Model file for the job. Use its own axes, mm. A direction names the side the tool comes from. Give positions to 0.01 mm unless a question says otherwise; leave off trailing zeros. Write each loop counter-clockwise with the first axis right and the second up, starting at its lowest first coordinate (ties: lowest second). Pieces come first, ordered by that corner, then holes. Notation, with made-up numbers: (86, -28) - (103, -28) arc R12 ccw to (103, -15) - close; hole circle Ø7 at (-10, -12.5). An arc over 180 degrees is marked (long way). One line per item, written item: value. Start each with the question number.
(1) 3-axis set-ups, long thin cutter, end or side, ignore diameter. For faces 5 (the face through (-2.685, -34.419, 0.426)), 6 (the face through (2.215, -24, 2)): which of +Z, -Z, +X, -X, +Y, -Y reach the whole face in a straight line?
(2) Cut at C-C, the plane y = -40.5. List the corners of the cut face in (x, z).
(3) Drop flat-ended pins along their axis: P1, Ø0.9, axis at y = -34.426, z = 1.5, coming from the -X side; P2, Ø1.4, axis at y = -14.426, z = 1.5, coming from the -X side. Give the stop position or say it passes through.
(4) Cut at B-B, the plane z = 0.35. State how many separate pieces and enclosed holes the cut face has, and give its area (3 significant figures).
(5) Probe L1, parallel to Y at x = -1.9, z = 1.5; L2, parallel to Y at x = 5, z = 1; L3, parallel to Y at x = -0.75, z = 1.9. List the from-to ranges inside material, lowest first.
(6) Cut at A-A, the plane y = -22. List the corners of the cut face in (x, z).
(7) Mould opens along Z. For faces 1 (the face through (1.904, -14.559, 1.471)), 2 (the face through (-2.785, -9, 1)), 3 (the face through (0, -24, 3)), 4 (the face through (-0.605, -35.203, 1.398)) say: pulls with the +Z half, pulls with the -Z half, needs draft (parallel to the pull), parting line crosses it, or undercut.
Autodesk Inventor part; units mm, degrees
ref_plane "YZ Plane" through (0, 0, 0) normal (1, 0, 0) x (0, 1, 0)
ref_plane "XZ Plane" through (0, 0, 0) normal (0, 1, 0) x (-1, 0, 0)
ref_plane "XY Plane" through (0, 0, 0) normal (0, 0, 1) x (1, 0, 0)
sketch "スケッチ1" plane through (0, 0, 0) normal (0, 0, 1) x (1, 0, 0)
  line L0 (22.7151, -43.926) -> (22.7151, -4.926) construction
  arc A0 (22.2151, -44.426) -> (22.7151, -43.926) centre (22.2151, -43.926) ccw construction
  line L1 (3.2151, -44.426) -> (22.2151, -44.426) construction
  arc A1 (2.7151, -43.926) -> (3.2151, -44.426) centre (3.2151, -43.926) ccw construction
  line L2 (2.7151, -4.926) -> (2.7151, -43.926) construction
  arc A2 (3.2151, -4.426) -> (2.7151, -4.926) centre (3.2151, -4.926) ccw construction
  line L3 (22.2151, -4.426) -> (3.2151, -4.426) construction
  arc A3 (22.7151, -4.926) -> (22.2151, -4.426) centre (22.2151, -4.926) ccw construction
  line L4 (6.2865, -24.2474) -> (6.2865, -30.6046) construction
  line L5 (6.2865, -30.6046) -> (10.1437, -30.6046) construction
  line L6 (10.1437, -30.6046) -> (10.1437, -24.2474) construction
  line L7 (10.1437, -24.2474) -> (6.2865, -24.2474) construction
  circle A4 centre (12.7151, -31.826) radius 1.1519 construction
  line L8 (19.1437, -24.2474) -> (15.2865, -24.2474) construction
  line L9 (15.2865, -24.2474) -> (15.2865, -30.6046) construction
  line L10 (15.2865, -30.6046) -> (19.1437, -30.6046) construction
  line L11 (19.1437, -30.6046) -> (19.1437, -24.2474) construction
  circle A5 centre (4.7151, -6.426) radius 1.8131 construction
  circle A6 centre (20.7151, -6.426) radius 1.8131 construction
  circle A7 centre (4.7151, -42.426) radius 1.8131 construction
  circle A8 centre (20.7151, -42.426) radius 1.8131 construction
  arc A9 (18.9651, -12.926) -> (6.4651, -12.9153) centre (12.7151, -12.926) ccw construction
  arc A10 (6.4649, -12.9153) -> (6.2151, -12.676) centre (6.2151, -12.926) ccw construction
  line L12 (6.2151, -12.676) -> (4.4651, -12.676) construction
  arc A11 (4.4651, -12.676) -> (4.4651, -13.176) centre (4.4651, -12.926) ccw construction
  line L13 (4.4651, -13.176) -> (6.2151, -13.176) construction
  arc A12 (6.2151, -13.176) -> (6.4651, -12.926) centre (6.2151, -12.926) ccw construction
  arc A13 (6.4651, -12.926) -> (6.9408, -15.3178) centre (12.7151, -12.926) ccw construction
  arc A14 (6.9408, -15.3178) -> (6.6142, -15.1825) centre (6.7099, -15.4134) ccw construction
  line L14 (6.6142, -15.1825) -> (4.9974, -15.8522) construction
  arc A15 (4.9974, -15.8522) -> (5.1888, -16.3141) centre (5.0931, -16.0831) ccw construction
  line L15 (5.1888, -16.3141) -> (6.8055, -15.6444) construction
  arc A16 (6.8055, -15.6444) -> (6.9408, -15.3178) centre (6.7099, -15.4134) ccw construction
  arc A17 (6.9408, -15.3178) -> (8.2957, -17.3454) centre (12.7151, -12.926) ccw construction
  arc A18 (8.2957, -17.3454) -> (7.9421, -17.3454) centre (8.1189, -17.5222) ccw construction
  line L16 (7.9421, -17.3454) -> (6.7047, -18.5829) construction
  arc A19 (6.7047, -18.5829) -> (7.0582, -18.9364) centre (6.8815, -18.7596) ccw construction
  line L17 (7.0582, -18.9364) -> (8.2957, -17.699) construction
  arc A20 (8.2957, -17.699) -> (8.2957, -17.3454) centre (8.1189, -17.5222) ccw construction
  arc A21 (8.2957, -17.3454) -> (10.3233, -18.7003) centre (12.7151, -12.926) ccw construction
  arc A22 (10.3233, -18.7003) -> (9.9967, -18.8356) centre (10.2277, -18.9312) ccw construction
  line L18 (9.9967, -18.8356) -> (9.327, -20.4523) construction
  arc A23 (9.327, -20.4523) -> (9.7889, -20.6437) centre (9.558, -20.548) ccw construction
  line L19 (9.7889, -20.6437) -> (10.4586, -19.0269) construction
  arc A24 (10.4586, -19.0269) -> (10.3233, -18.7003) centre (10.2277, -18.9312) ccw construction
  arc A25 (10.3233, -18.7003) -> (12.7151, -19.176) centre (12.7151, -12.926) ccw construction
  arc A26 (12.7151, -19.176) -> (12.4651, -19.426) centre (12.7151, -19.426) ccw construction
  line L20 (12.4651, -19.426) -> (12.4651, -21.176) construction
  arc A27 (12.4651, -21.176) -> (12.9651, -21.176) centre (12.7151, -21.176) ccw construction
  line L21 (12.9651, -21.176) -> (12.9651, -19.426) construction
  arc A28 (12.9651, -19.426) -> (12.7151, -19.176) centre (12.7151, -19.426) ccw construction
  arc A29 (12.7151, -19.176) -> (15.1069, -18.7003) centre (12.7151, -12.926) ccw construction
  arc A30 (15.1069, -18.7003) -> (14.9716, -19.0269) centre (15.2025, -18.9312) ccw construction
  line L22 (14.9716, -19.0269) -> (15.6413, -20.6437) construction
  arc A31 (15.6413, -20.6437) -> (16.1032, -20.4523) centre (15.8722, -20.548) ccw construction
  line L23 (16.1032, -20.4523) -> (15.4335, -18.8356) construction
  arc A32 (15.4335, -18.8356) -> (15.1069, -18.7003) centre (15.2025, -18.9312) ccw construction
  arc A33 (15.1069, -18.7003) -> (17.1345, -17.3454) centre (12.7151, -12.926) ccw construction
  arc A34 (17.1345, -17.3454) -> (17.1345, -17.699) centre (17.3113, -17.5222) ccw construction
  line L24 (17.1345, -17.699) -> (18.3719, -18.9364) construction
  arc A35 (18.3719, -18.9364) -> (18.7255, -18.5829) centre (18.5487, -18.7596) ccw construction
  line L25 (18.7255, -18.5829) -> (17.4881, -17.3454) construction
  arc A36 (17.4881, -17.3454) -> (17.1345, -17.3454) centre (17.3113, -17.5222) ccw construction
  arc A37 (17.1345, -17.3454) -> (18.4893, -15.3178) centre (12.7151, -12.926) ccw construction
  arc A38 (18.4893, -15.3178) -> (18.6246, -15.6444) centre (18.7203, -15.4134) ccw construction
  line L26 (18.6246, -15.6444) -> (20.2414, -16.3141) construction
  arc A39 (20.2414, -16.3141) -> (20.4328, -15.8522) centre (20.3371, -16.0831) ccw construction
  line L27 (20.4328, -15.8522) -> (18.816, -15.1825) construction
  arc A40 (18.816, -15.1825) -> (18.4893, -15.3178) centre (18.7203, -15.4134) ccw construction
  arc A41 (18.4893, -15.3178) -> (18.9651, -12.926) centre (12.7151, -12.926) ccw construction
  arc A42 (18.9651, -12.926) -> (19.2151, -13.176) centre (19.2151, -12.926) ccw construction
  line L28 (19.2151, -13.176) -> (20.9651, -13.176) construction
  arc A43 (20.9651, -13.176) -> (20.9651, -12.676) centre (20.9651, -12.926) ccw construction
  line L29 (20.9651, -12.676) -> (19.2151, -12.676) construction
  arc A44 (19.2151, -12.676) -> (18.9651, -12.926) centre (19.2151, -12.926) ccw construction
  circle A45 centre (4.7151, -6.426) radius 1.1
  circle A46 centre (4.7151, -42.426) radius 1.1
  circle A47 centre (4.7151, -6.426) radius 2.5
  circle A48 centre (4.7151, -42.426) radius 2.5
  circle A49 centre (12.7151, -12.926) radius 8 construction
  circle A50 centre (12.7151, -12.926) radius 8
  line L30 (12.1437, -22.2474) -> (12.1437, -32.6046)
  line L31 (12.1437, -32.6046) -> (4.2865, -32.6046)
  line L32 (4.2865, -32.6046) -> (4.2865, -22.2474)
  line L33 (4.2865, -22.2474) -> (12.1437, -22.2474)
  line L34 (7.2151, -6.426) -> (7.2151, -42.426)
  line L35 (4.7151, -3.926) -> (-2.7849, -3.926)
  line L36 (-2.7849, -3.926) -> (-2.7849, -44.926)
  line L37 (-2.7849, -44.926) -> (4.7151, -44.926)
  circle A51 centre (-3.7849, -14.426) radius 1.1
  line L38 (7.2151, -24.426) -> (-2.7849, -24.426) construction
  circle A52 centre (-3.7849, -34.426) radius 1.1
  point P0 (0, 0)
  point P1 (7.0743, -7.2531)
  point P2 (-2.7849, -13.9677)
  point P3 (-2.7849, -14.8843)
  point P4 (-2.7849, -33.9677)
  point P5 (-2.7849, -34.8843)
  point P6 (7.2151, -32.6046)
  point P7 (7.2151, -22.2474)
  point P8 (7.2151, -18.7355)
  point P9 (7.2151, -7.1165)
  dimension "d0" = 2.2
  dimension "d1" = 2.2
  dimension "d3" = 5
  dimension "d4" = 5
  dimension "d5" = 2
  dimension "d6" = 10
  dimension "d7" = 2.2
  dimension "d8" = 1
  dimension "d9" = 10
extrude "押し出し1" add sketch "スケッチ1" along normal blind 3 contours A47 A50 | L34 A50 A47 | A47 A50 L34 L33 L32 L31 A48 L37 L36 A52 A51 L35 | A48 picked at (5.5204, -8.2788) picked at (7.1889, -6.9354)
fillet "フィレット1" radius 2 4 edges at (7.2151, -22.2474, 1.5) (7.2151, -32.6046, 1.5) (4.2865, -32.6046, 1.5) (4.2865, -22.2474, 1.5)
sketch "スケッチ2" plane through (-2.7849, -33.9677, 0) normal (-1, 0, 0) x (0, 0, 1)
  line L0 (0, 20) -> (3, 20)
  line L1 (3, 20) -> (3, 19.0835)
  line L2 (3, 0) -> (3, -0.9165)
  point P0 (0, 33.9677)
  point P1 (1.5, 19.5417)
  point P2 (1.5, 20)
  point P3 (3, 19.5417)
  point P4 (1.5, -0.4583)
  point P5 (3, -0.4583)
hole "穴1" at (-2.7849, -14.426, 1.5) at (-2.7849, -34.426, 1.5) direction (1, 0, 0) diameter 1.567 depth 4.3 tip angle 118
sketch "スケッチ3" plane through (0, 0, 3) normal (0, 0, 1) x (1, 0, 0)
  circle A0 centre (4.7151, -6.426) radius 1.1
  arc A1 (7.2151, -6.426) -> (4.7151, -3.926) centre (4.7151, -6.426) ccw
  circle A2 centre (4.7151, -42.426) radius 1.1
  arc A3 (4.7151, -44.926) -> (7.2151, -42.426) centre (4.7151, -42.426) ccw
  circle A4 centre (4.7151, -42.426) radius 2.5
  line L0 (4.7151, -8.926) -> (2.2151, -8.926)
  line L1 (2.2151, -8.926) -> (2.2151, -39.926)
  line L2 (2.2151, -39.926) -> (4.7151, -39.926)
  line L3 (-2.7849, -3.926) -> (-2.7849, -44.926)
  arc A5 (5.7508, -22.1743) -> (7.2151, -20.2474) centre (5.2151, -20.2474) ccw
  line L4 (7.2151, -20.2474) -> (7.2151, -18.7355)
  arc A6 (7.2151, -6.426) -> (4.7151, -3.926) centre (4.7151, -6.426) ccw
  line L5 (4.7151, -3.926) -> (-2.7849, -3.926)
  line L6 (-2.7849, -3.926) -> (-2.7849, -13.9677)
  line L7 (-2.7849, -44.926) -> (4.7151, -44.926)
  arc A7 (4.7151, -44.926) -> (7.2151, -42.426) centre (4.7151, -42.426) ccw
  line L8 (7.2151, -42.426) -> (7.2151, -34.6046)
  arc A8 (7.2151, -34.6046) -> (5.7508, -32.6777) centre (5.2151, -34.6046) ccw
  circle A9 centre (4.7151, -42.426) radius 1.1
  circle A10 centre (4.7151, -6.426) radius 1.1
  line L9 (4.2865, -30.7508) -> (4.2865, -24.1012)
  arc A11 (5.7508, -22.1743) -> (4.2865, -24.1012) centre (6.2865, -24.1012) ccw
  arc A12 (4.2865, -30.7508) -> (5.7508, -32.6777) centre (6.2865, -30.7508) ccw
  arc A13 (-2.7849, -14.8843) -> (-2.7849, -13.9677) centre (-3.7849, -14.426) ccw
  line L10 (-2.7849, -14.8843) -> (-2.7849, -33.9677)
  arc A14 (-2.7849, -34.8843) -> (-2.7849, -33.9677) centre (-3.7849, -34.426) ccw
  line L11 (-2.7849, -34.8843) -> (-2.7849, -44.926)
  circle A15 centre (4.7151, -6.426) radius 2.5
  arc A16 (7.2151, -7.1165) -> (7.2151, -18.7355) centre (12.7151, -12.926) ccw
  line L12 (7.2151, -7.1165) -> (7.2151, -6.426)
  point P0 (0, 0)
  point P1 (7.0743, -7.2531)
  point P2 (-2.7849, -14.8843)
  point P3 (-2.7849, -34.8843)
  point P4 (7.0743, -7.2531)
  point P5 (6.0077, -8.5659)
  dimension "d20" = 5
extrude "押し出し2" cut sketch "スケッチ3" against normal through all contours A0 | L12 A16 A15 | A15 A16 L4 A5 A11 L9 A12 A8 L8 A4 L2 L1 L0 | A13 L3 | A14 L3
fillet "フィレット2" radius 4 2 edges at (2.2151, -8.926, 1.5) (2.2151, -39.926, 1.5)
fillet "フィレット3" radius 4 1 edges at (6.0077, -8.5659, 1.5)
properties part number "asikubi_asi" material "アルミニウム 2014-T4"
Answers follow:
1. face 5: +Z, -Z, -X
1. face 6: +Z, -Z, +X
2. outline: (-2.78, 0) - (6.31, 0) - (6.31, 3) - (-2.78, 3) - close
3. P1: stops at x = 1.72
3. P2: stops at x = 1.57
4. separate pieces: 1
4. enclosed holes: 2
4. area: 247 mm²
5. L1: y = -44.93 to -35.21, -33.64 to -15.21, -13.64 to -3.93
5. L2: y = -44.91 to -43.49, -41.36 to -39.91, -8.93 to -7.49, -5.36 to -3.94
5. L3: y = -44.93 to -35.1, -33.75 to -15.1, -13.75 to -3.93
6. outline: (-2.78, 0) - (2.22, 0) - (2.22, 3) - (-2.78, 3) - close
7. face 1: undercut
7. face 2: needs draft
7. face 3: pulls with the +Z half
7. face 4: undercut
